from build123d import *

# Parameters (mm, degrees)
F6_DEPTH        = 21
F7_SIZE         = 2
F8_SIZE         = 2
F12_DEPTH       = 2.5510001
F14_D           = 2.5
F14_CSINK_D     = 4
F14_CSINK_ANGLE = 90


# Not quite as in the source:
# - a feature names something its author has since deleted; it is built from what else it names


with BuildPart() as f6:
    # F5 (on Front) → F6 (new body)
    with BuildSketch(Plane.XZ):
        with BuildLine():
            ThreePointArc((1.75, 6.2599920128), (3.3753918927, 5.5548833985), (4.75, 4.4370598373))
            Line((4.75, 4.4370598373), (4.75, 9.2370598373))
            Line((4.75, 9.2370598373), (-4.75, 9.2370598373))
            Line((-4.75, 9.2370598373), (-4.75, 4.4370598373))
            ThreePointArc((-4.75, 4.4370598373), (-3.3753918927, 5.5548833985), (-1.75, 6.2599920128))
            Line((-1.75, 6.2599920128), (-1.75, 6.9870598373))
            ThreePointArc((-1.75, 6.9870598373), (0, 8.7370598373), (1.75, 6.9870598373))
            Line((1.75, 6.9870598373), (1.75, 6.2599920128))
        make_face()
        with BuildLine():
            ThreePointArc((-1.75, 6.2599920128), (0, 6.5), (1.75, 6.2599920128))
            Line((1.75, 6.2599920128), (1.75, 6.9870598373))
            ThreePointArc((1.75, 6.9870598373), (0, 8.7370598373), (-1.75, 6.9870598373))
            Line((-1.75, 6.9870598373), (-1.75, 6.2599920128))
        make_face()
    extrude(amount=-F6_DEPTH)

    # F7
    f7_edges = [f6.edges().sort_by_distance(p)[0] for p in [
        (-4.75, 10.5, 9.23706),
        (4.75, 10.5, 9.23706),
    ]]
    chamfer(f7_edges, length=F7_SIZE)

    # F8
    f8_edges = [f6.edges().sort_by_distance(p)[0] for p in [
        (0, 21, 9.23706),
    ]]
    chamfer(f8_edges, length=F8_SIZE)

    # F10 (on offset) → F11 (revolve, cut)
    with BuildSketch(Plane.XY.offset(6.9870598373)):
        with BuildLine():
            Line((-1.75, 11.75), (-1.75, 0))
            Line((-1.75, 0), (0, 0))
            Line((0, 0), (0, 13.5))
            ThreePointArc((0, 13.5), (-1.2374368671, 12.9874368671), (-1.75, 11.75))
        make_face()
    revolve(axis=Axis((0, 6.75, 6.9870598373), (0, 1, 0)), mode=Mode.SUBTRACT)

    # F10 (on offset) → F12 (cut, through all)
    with BuildSketch(Plane.XY.offset(6.9870598373)):
        with BuildLine():
            Line((0, 13.5), (0, 0))
            Line((0, 0), (1.75, 0))
            Line((1.75, 0), (1.75, 11.75))
            ThreePointArc((1.75, 11.75), (1.2374368671, 12.9874368671), (0, 13.5))
        make_face()
        with BuildLine():
            Line((-1.75, 11.75), (-1.75, 0))
            Line((-1.75, 0), (0, 0))
            Line((0, 0), (0, 13.5))
            ThreePointArc((0, 13.5), (-1.2374368671, 12.9874368671), (-1.75, 11.75))
        make_face()
    extrude(amount=-F12_DEPTH, mode=Mode.SUBTRACT)

    # F14 (through all)
    with Locations(Plane.XY.offset(9.2370598373)):
        with Locations((0, 16)):
            CounterSinkHole(F14_D / 2, F14_CSINK_D / 2, counter_sink_angle=F14_CSINK_ANGLE)


solid = f6.part
Check sheet for the modelled part. Datum: model origin and axes. Units: mm. Round coordinates to 2 decimals unless told otherwise and drop trailing zeros. Order: outer loops, then holes, each group sorted by start corner. A loop starts at its lowest first (then second) coordinate and runs counter-clockwise, first axis right, second up.
Q1. Draft check along X on faces 1 (the face through (-3.764, 10.353, 8.223)), 2 (the face through (0, 9, 9.237)), 3 (the face through (-0.038, 5.793, 8.737)). Enter one of: pulls with the +X half, pulls with the -X half, needs draft (parallel to the pull), parting line crosses it, or undercut.
Filled sheet:
face 1: pulls with the -X half
face 2: needs draft
face 3: undercut
Q2. Cross-section at D-D, the plane x = -3. Enter the section's corners in (y, z).
Filled sheet:
outline: (0, 5.77) - (21, 5.77) - (21, 7.24) - (19.25, 8.99) - (0, 8.99) - close
Q3. Depth check by flat-ended pin: P1, Ø2, axis at x = 0, y = 16, coming from the -Z side; P2, Ø4, axis at x = 2, y = 14, coming from the -Z side. Enter the tip coordinate at first touch or a pass-through.
Filled sheet:
P1: passes through
P2: stops at z = 5.12
Q4. Cross-section at C-C, the plane y = 11.25. Enter the section's corners in (x, z).
Filled sheet:
outline: (-4.75, 4.44) arc R6.5 cw to (-1.75, 6.26) - (-1.75, 6.99) arc R1.75 cw to (1.75, 6.99) - (1.75, 6.26) arc R6.5 cw to (4.75, 4.44) - (4.75, 7.24) - (2.75, 9.24) - (-2.75, 9.24) - (-4.75, 7.24) - close
Q5. Scan lines: L1, parallel to X at y = 16, z = 6.85; L2, parallel to X at y = 11, z = 6.3; L3, parallel to Y at x = 0, z = 7.5. Record each from-to range of solid material in increasing order.
Filled sheet:
L1: x = -4.75 to -1.25, 1.25 to 4.75
L2: x = -4.75 to -1.75, 1.75 to 4.75
L3: y = 13.42 to 14.75, 17.25 to 20.74
Q6. Cross-section at B-B, the plane z = 5.8. Enter the section's corners in (x, y).
Filled sheet:
outline: (-4.75, 0) - (-2.93, 0) - (-2.93, 21) - (-4.75, 21) - close; (2.93, 0) - (4.75, 0) - (4.75, 21) - (2.93, 21) - close
Q7. Cross-section at A-A, the plane y = 16. Enter the section's corners in (x, z), plus the area to 3 significant figures.
Filled sheet:
outline: (-4.75, 4.44) arc R6.5 cw to (-1.25, 6.38) - (-1.25, 8.49) - (-2, 9.24) - (-2.75, 9.24) - (-4.75, 7.24) - close; (1.25, 6.38) arc R6.5 cw to (4.75, 4.44) - (4.75, 7.24) - (2.75, 9.24) - (2, 9.24) - (1.25, 8.49) - close
area: 20.5 mm2
